Geometry check sheet. Reference: the model listing, model coordinates, mm. Face numbers are marked on the shaded views. A direction names the side the tool comes from. Round coordinates to 2 decimals unless told otherwise and drop trailing zeros. Loops run counter-clockwise (first coordinate to the right, second up) from the corner with the lowest first, then second, coordinate; pieces in that order, holes last. Notation, with made-up numbers: (-5, 74.5) -> (52, 74.5) arc R8 ccw to (52, 88.5) -> close; hole circle Ø5 at (31, 56). An arc over 180 degrees is marked (long way). Use one line per item in the form item = value.
Autodesk Inventor part; units mm, degrees
ref_plane "YZ Plane" through (0, 0, 0) normal (1, 0, 0) x (0, 1, 0)
ref_plane "XZ Plane" through (0, 0, 0) normal (0, 1, 0) x (-1, 0, 0)
ref_plane "XY Plane" through (0, 0, 0) normal (0, 0, 1) x (1, 0, 0)
sketch "Sketch1" plane through (0, 0, 0) normal (0, 1, 0) x (-1, 0, 0)
  line L0 (0, 0) -> (38.1, 0)
  line L1 (38.1, 0) -> (38.1, -38.1)
  line L2 (38.1, -38.1) -> (0, -38.1)
  line L3 (0, -38.1) -> (0, 0)
  dimension "d0" = 38.1
  dimension "d1" = 38.1
extrude "Extrusion1" add sketch "Sketch1" along normal blind 3.81
sketch "Sketch2" plane through (0, 3.81, 0) normal (0, 1, 0) x (1, 0, 0)
  line L0 (-38.1, 0) -> (0, 0)
  line L1 (0, 0) -> (0, 38.1)
  line L2 (0, 38.1) -> (-38.1, 38.1)
  line L3 (-38.1, 38.1) -> (-38.1, 0)
  line L4 (-38.1, 0) -> (0, 0)
  line L5 (0, 0) -> (0, -11.8097)
  line L6 (0, -11.8097) -> (-38.1, -11.8097)
  line L7 (-38.1, -11.8097) -> (-38.1, 0)
  line L8 (-38.1, 38.1) -> (0, 38.1)
  line L9 (0, 38.1) -> (0, 49.9227)
  line L10 (0, 49.9227) -> (-38.1, 49.9227)
  line L11 (-38.1, 49.9227) -> (-38.1, 38.1)
extrude "Extrusion2" add sketch "Sketch2" along normal blind 3.81
sketch "Sketch3" plane through (0, 7.62, 0) normal (0, 1, 0) x (1, 0, 0)
  line L0 (-38.1, -11.8097) -> (0, -11.8097)
  line L1 (-19.05, -11.8097) -> (-19.05, -5.7137)
  line L2 (0, 49.9227) -> (-38.1, 49.9227)
  line L3 (-19.05, 49.9227) -> (-19.05, 43.8267)
  circle A0 centre (-19.05, -5.7137) radius 3.048
  circle A1 centre (-19.05, 43.8267) radius 3.048
  point P0 (0, 0)
  dimension "d6" = 6.096
  dimension "d7" = 6.096
  dimension "d8" = 6.096
extrude "Extrusion3" cut sketch "Sketch3" against normal blind 3.81
properties part number "peltier and mount" material "Aluminum 6061-AHC"
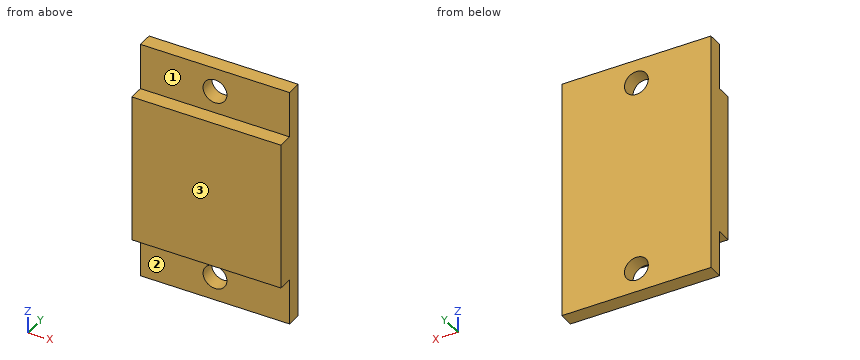
1. Section check D-D (y = 4.75). Record the boundary of the cut face in (x, z), then the cut area to 3 significant figures.
Return value:
outline = (-38.1, -49.92) -> (0, -49.92) -> (0, 11.81) -> (-38.1, 11.81) -> close; hole circle Ø6.1 at (-19.05, -43.83); hole circle Ø6.1 at (-19.05, 5.71)
area = 2,290 mm2
2. Section check B-B (z = 8). Record the boundary of the cut face in (x, y), then the cut area to 3 significant figures.
Return value:
outline = (-38.1, 3.81) -> (-21.07, 3.81) -> (-21.07, 7.62) -> (-38.1, 7.62) -> close; (-17.03, 3.81) -> (0, 3.81) -> (0, 7.62) -> (-17.03, 7.62) -> close
area = 130 mm2
3. Gauge pin test, flat ends, axial feed: pin 1 (1.9 mm diameter, centred on x = -13.5, y = 2, fed in from +Z); pin 2 (2 mm diameter, centred on x = -23, y = 1, fed in from -Z); pin 3 (6 mm diameter, centred on x = -17, z = 4, fed in from -Y). Record the tip position at first contact, or that the pin passes through.
Return value:
pin_1 = 0
pin_2 = -38.1
pin_3 = 3.81
4. Tool access check on the marked faces 1, 2 and 3. Record the directions out of +Z, -Z, +X, -X, +Y, -Y that give a thin tool (end or side, any length) a straight path to the whole face; none if there is none.
Return value:
face_1 = +Z, +X, -X, -Y
face_2 = -Z, +X, -X, -Y
face_3 = +Z, -Z, +X, -X, -Y
5. Section check A-A (x = -19.05). Record the boundary of the cut face in (y, z).
Return value:
outline = (0, -38.1) -> (3.81, -38.1) -> (3.81, -40.78) -> (7.62, -40.78) -> (7.62, 2.67) -> (3.81, 2.67) -> (3.81, 0) -> (0, 0) -> close; (3.81, -49.92) -> (7.62, -49.92) -> (7.62, -46.87) -> (3.81, -46.87) -> close; (3.81, 8.76) -> (7.62, 8.76) -> (7.62, 11.81) -> (3.81, 11.81) -> close
6. Material ranges on line 1 along Z through (x, y) = (-19.05, 5.2); line 2 along Y through (x, z) = (-31, 5); line 3 along Z through (x, y) = (-34, 3), recorded low to high.
Return value:
line_1 = -49.92 to -46.87, -40.78 to 2.67, 8.76 to 11.81
line_2 = 3.81 to 7.62
line_3 = -38.1 to 0
7. Section check C-C (x = -11.5). Record the boundary of the cut face in (y, z), then the cut area to 3 significant figures.
Return value:
outline = (0, -38.1) -> (3.81, -38.1) -> (3.81, -49.92) -> (7.62, -49.92) -> (7.62, 11.81) -> (3.81, 11.81) -> (3.81, 0) -> (0, 0) -> close
area = 380 mm2
